Source: three-view drawing plus pictorial views. Frame: mm from the lowest corner of the part. A direction names the side the tool comes from. Give positions to 0.01 mm unless a question says otherwise; leave off trailing zeros. Write each loop counter-clockwise with the first axis right and the second up, starting at its lowest first coordinate (ties: lowest second). Pieces come first, ordered by that corner, then holes. Notation, with made-up numbers: M -20,39 L -13,39 A27 ccw -13,65 Z; hole C -13.5,-6 d7. An arc over 180 degrees is marked long. Return JSON: item names as keys, results as strings.
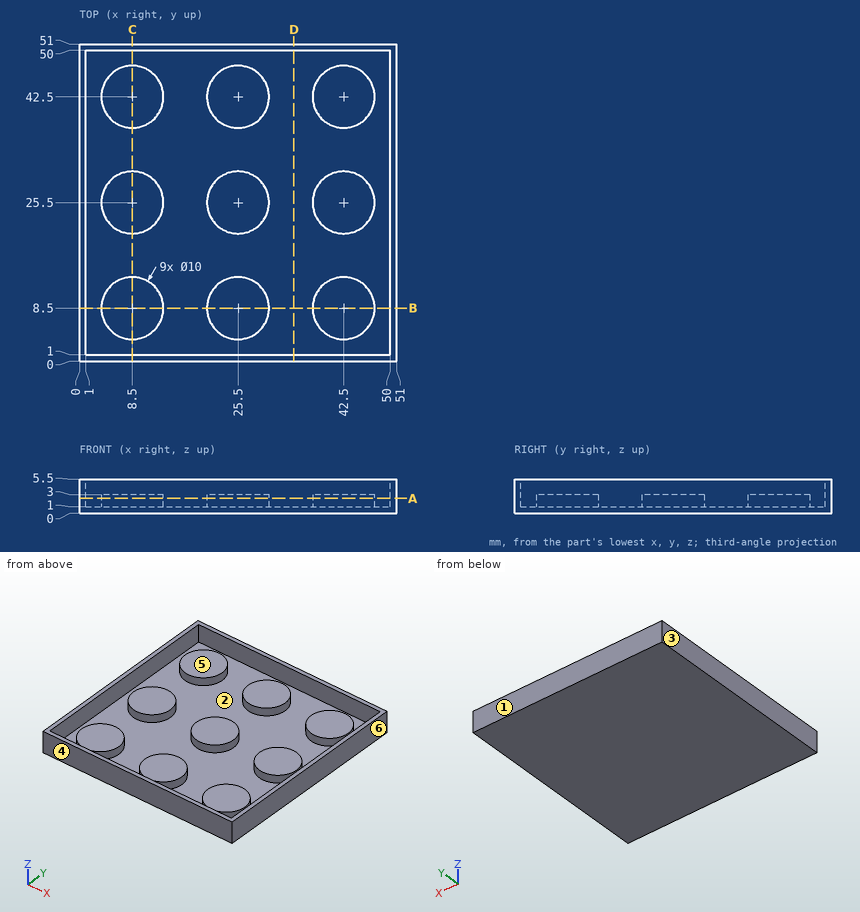
1) Line query: line 1 (X direction, y = 19, z = 3.7); line 2 (X direction, y = 29, z = 2.5). Output: solid intervals per line, ascending. Write a range as [from, to].
Numbers:
{"line 1": "x = [0, 1], [50, 51]", "line 2": "x = [0, 1], [4.93, 12.07], [21.93, 29.07], [38.93, 46.07], [50, 51]"}
2) Cut plane A-A, the plane z = 2.4. Give the number of separate pieces and of enclosed holes in the cut face, then the cut area to 3 significant figures.
Numbers:
{"separate pieces": "10", "enclosed holes": "1", "area": "907 mm²"}
3) Set-up query: the marked faces 5 and 6. Return all of +Z, -Z, +X, -X, +Y, -Y with unobstructed straight access to the full face (end or side cutting, diameter ignored); none if empty.
Numbers:
{"face 5": "+Z", "face 6": "+Z, -Z, +X, +Y, -Y"}
4) Cut plane B-B, the plane y = 8.5. Return the cut outline in (x, z).
Numbers:
{"outline": "M 0,0 L 51,0 L 51,5.5 L 50,5.5 L 50,1 L 47.5,1 L 47.5,3 L 37.5,3 L 37.5,1 L 30.5,1 L 30.5,3 L 20.5,3 L 20.5,1 L 13.5,1 L 13.5,3 L 3.5,3 L 3.5,1 L 1,1 L 1,5.5 L 0,5.5 Z"}
5) Draft query along Y for the marked faces 1, 2, 3 and 4. Return one class per face: released by +Y, released by -Y, zero draft, split by the parting line, or undercut.
Numbers:
{"face 1": "released by +Y", "face 2": "undercut", "face 3": "zero draft", "face 4": "released by -Y"}
6) Cut plane D-D, the plane x = 34.5. Return the cut outline in (y, z).
Numbers:
{"outline": "M 0,0 L 51,0 L 51,5.5 L 50,5.5 L 50,1 L 1,1 L 1,5.5 L 0,5.5 Z"}
7) Contact query for a flat-ended pin moving along its axis: pin 1 Ø8 at (x, y) = (28, 42.5) entering from +Z. Output: stop coordinate, or through.
Numbers:
{"pin 1": "stops at z = 3"}
